Part model, mm, in its own coordinate system. Face numbers are marked on the shaded views. A direction names the side the tool comes from. Give positions to 0.01 mm unless a question says otherwise; leave off trailing zeros. Write each loop counter-clockwise with the first axis right and the second up, starting at its lowest first coordinate (ties: lowest second). Pieces come first, ordered by that corner, then holes. Notation, with made-up numbers: M 35,-38 L 72,-38 A14 cw 72,-29 Z; hole C 70.5,5.25 d9. An arc over 180 degrees is marked long. Answer as CSV lines item,"result". Start each with the question number.
Item 1: 3-axis set-ups, long thin cutter, end or side, ignore diameter. For the marked faces 1, 2 and 3: which of +Z, -Z, +X, -X, +Y, -Y reach the whole face in a straight line?
Item 2: Band-saw the part on C-C, the plane z = 8. List the corners of the cut face in (x, y) (3 decimals).
Item 3: Band-saw the part on D-D, the plane y = 23.5. List the corners of the cut face in (x, z).
Item 4: Pin check, flat tips, straight feed: pin 1 (7 mm diameter, centred on y = 22.5, z = 4, fed in from +X); pin 2 (3 mm diameter, centred on x = 4, z = 10, fed in from +Y); pin 3 (4 mm diameter, centred on y = 46, z = 1.5, fed in from -X). Stop position of each tip, or through.
Item 5: Band-saw the part on B-B, the plane x = 0. Count the separate pieces of the cut face and the enclosed holes in it, then the cut area to 3 significant figures.
Item 6: Wall check: L1, parallel to Y at x = 0, z = 4.75; L2, parallel to Y at x = 0, z = 8.75 (3 decimals); L3, parallel to X at y = 12.7, z = 3.5. Give the ranges that are in metal, low to high. Write a range as from..to.
from build123d import *

# Parameters (mm, degrees)
F1_DEPTH       = 6.35
F2_R           = 3.175
F3_DEPTH       = 6.35
F5_D           = 2.032
F5_CSINK_D     = 3.175
F5_CSINK_ANGLE = 82
F7_D           = 2.032
F7_CSINK_D     = 3.175
F7_CSINK_ANGLE = 82


with BuildPart() as f1:
    # F0 (on Top) → F1 (new body)
    with BuildSketch(Plane.XY):
        with BuildLine():
            ThreePointArc((-5.08, 12.7), (-3.5921024484, 9.1078975516), (0, 7.62))
            Line((0, 7.62), (0, 12.7))
            Line((0, 12.7), (0, 17.78))
            ThreePointArc((0, 17.78), (-3.5921024484, 16.2921024484), (-5.08, 12.7))
        make_face()
        with BuildLine():
            Line((0, 12.7), (0, 7.62))
            ThreePointArc((0, 7.62), (3.5921024484, 9.1078975516), (5.08, 12.7))
            ThreePointArc((5.08, 12.7), (3.5921024484, 16.2921024484), (0, 17.78))
            Line((0, 17.78), (0, 12.7))
        make_face()
        with BuildLine():
            ThreePointArc((5.08, 12.7), (3.5921024484, 9.1078975516), (0, 7.62))
            ThreePointArc((0, 7.62), (-3.5921024484, 9.1078975516), (-5.08, 12.7))
            Line((-5.08, 12.7), (-5.08, 0))
            ThreePointArc((-5.08, 0), (0, -5.08), (5.08, 0))
            Line((5.08, 0), (5.08, 12.7))
        make_face()
        with BuildLine():
            ThreePointArc((0, 17.78), (3.5921024484, 16.2921024484), (5.08, 12.7))
            Line((5.08, 12.7), (5.08, 32.7368881382))
            Line((5.08, 32.7368881382), (4.2115108686, 31.4493000504))
            ThreePointArc((4.2115108686, 31.4493000504), (2.384915539, 29.8046262283), (0, 29.21))
            Line((0, 29.21), (0, 17.78))
        make_face()
        with BuildLine():
            Line((-5.08, 34.29), (-5.08, 12.7))
            ThreePointArc((-5.08, 12.7), (-3.5921024484, 16.2921024484), (0, 17.78))
            Line((0, 17.78), (0, 29.21))
            ThreePointArc((0, 29.21), (-3.5921024484, 30.6978975516), (-5.08, 34.29))
        make_face()
        with BuildLine():
            Line((5.08, 34.29), (5.08, 32.7368881382))
            Line((5.08, 32.7368881382), (26.9371104656, 65.141386999))
            ThreePointArc((26.9371104656, 65.141386999), (25.5662995467, 72.1935978172), (18.5140887285, 70.8227868983))
            Line((18.5140887285, 70.8227868983), (-4.2115108686, 37.1306999496))
            ThreePointArc((-4.2115108686, 37.1306999496), (-0.9693096965, 39.2766660919), (2.8406999496, 38.5015108686))
            ThreePointArc((2.8406999496, 38.5015108686), (4.4853737717, 36.674915539), (5.08, 34.29))
        make_face()
        with BuildLine():
            Line((4.2115108686, 31.4493000504), (5.08, 32.7368881382))
            Line((5.08, 32.7368881382), (5.08, 34.29))
            ThreePointArc((5.08, 34.29), (4.4853737717, 36.674915539), (2.8406999496, 38.5015108686))
            Line((2.8406999496, 38.5015108686), (0, 34.29))
            Line((0, 34.29), (0, 29.21))
            ThreePointArc((0, 29.21), (2.384915539, 29.8046262283), (4.2115108686, 31.4493000504))
        make_face()
        with BuildLine():
            ThreePointArc((-4.2115108686, 37.1306999496), (-4.8580281603, 35.77524826), (-5.08, 34.29))
            ThreePointArc((-5.08, 34.29), (-3.5921024484, 30.6978975516), (0, 29.21))
            Line((0, 29.21), (0, 34.29))
            Line((0, 34.29), (2.8406999496, 38.5015108686))
            ThreePointArc((2.8406999496, 38.5015108686), (-0.9693096965, 39.2766660919), (-4.2115108686, 37.1306999496))
        make_face()
    extrude(amount=F1_DEPTH)

    # F2 (on face) → F3 (join)
    with BuildSketch(Plane.XY.offset(6.35)):
        with Locations((0, 12.7)):
            Circle(F2_R)
    extrude(amount=F3_DEPTH)

    # F5 (through all)
    with Locations(Plane.XY.offset(12.7)):
        with Locations((0, 12.7)):
            CounterSinkHole(F5_D / 2, F5_CSINK_D / 2, counter_sink_angle=F5_CSINK_ANGLE)

    # F7 (through all)
    with Locations(Plane.XY.offset(6.35)):
        with Locations((0, 0)):
            CounterSinkHole(F7_D / 2, F7_CSINK_D / 2, counter_sink_angle=F7_CSINK_ANGLE)


solid = f1.part
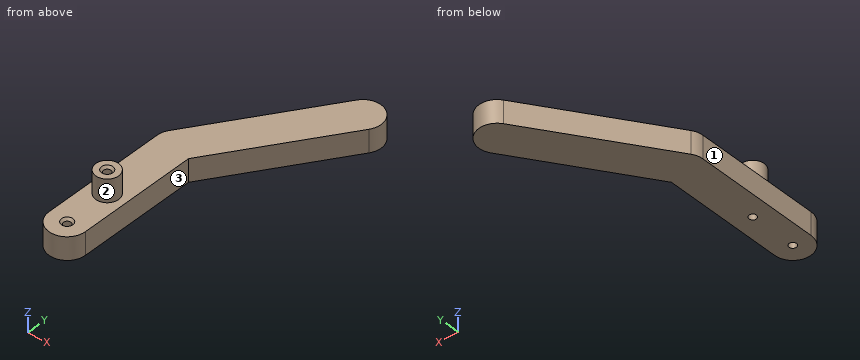
Output:
1,face 1,"+Z, -Z, -X, +Y, -Y"
1,face 2,"+Z"
1,face 3,"+Z, -Z, +X, -Y"
2,outline,"C 0,12.7 d6.35; hole C 0,12.7 d2.032"
3,outline,"M -5.08,0 L 5.08,0 L 5.08,6.35 L -5.08,6.35 Z"
4,pin 1,"x = 5.08"
4,pin 2,"y = 14.66"
4,pin 3,"x = 0.42"
5,separate pieces,"3"
5,enclosed holes,"0"
5,area,"309 mm²"
6,L1,"-5.08..-1.02, 1.02..11.68, 13.72..43.37"
6,L2,"9.525..11.684, 13.716..15.875"
6,L3,"-5.08..-1.02, 1.02..5.08"
